Verification items for the finished model (mm, model axes). A direction names the side the tool comes from. Give positions to 0.01 mm unless a question says otherwise; leave off trailing zeros. Order: outer loops, then holes, each group sorted by start corner. A loop starts at its lowest first (then second) coordinate and runs counter-clockwise, first axis right, second up. Notation, with made-up numbers: (62, 82.25) -> (104, 82.25) arc R14 ccw to (104, 106.25) -> close; hole circle Ø5 at (61, 42). An arc over 180 degrees is marked (long way). Return JSON: item names as keys, results as strings. Group by question number.
(1) Cross-section at A-A on x = 17.5. Enter the section's corners in (y, z).
(2) Cross-section at B-B on y = 8. Enter the section's corners in (x, z).
(3) Thickness scan on line 1 along Z through (x, y) = (18.5, 10); line 2 along Z through (x, y) = (16, -9). Record the ranges inside material, lowest first.
(4) Tool access check on faces 1 (the face through (0, 3.134, 61)), 2 (the face through (0, -3.134, 61)), 3 (the face through (0, -18.474, 1)). Record the directions out of +Z, -Z, +X, -X, +Y, -Y that give a thin tool (end or side, any length) a straight path to the whole face; none if there is none.
(5) Depth check by flat-ended pin: pin 1 Ø8 at (y, z) = (12, 54) entering from +X; pin 2 Ø5 at (x, z) = (-4, 40.5) entering from +Y; pin 3 Ø14 at (x, z) = (-11, 60.5) entering from +Y; pin 4 Ø14 at (x, z) = (1.5, 60) entering from -Y. Enter the tip coordinate at first touch or a pass-through.
(6) Cross-section at C-C on z = 41. Enter the section's corners in (x, y), then the cut area to 3 significant figures.
from build123d import *

# Parameters (mm, degrees)
F1_DEPTH      = 25.4
F1_DEPTH_BACK = 25.4


with BuildPart() as f1:
    # F0 (on Right) → F1 (new body, two sides)
    with BuildSketch(Plane.YZ) as f1_sk:
        Polygon((-18.474095, -38.079124), (18.474095, -38.079124), (18.474095, 38.079124), (3.134074, 54.85357), (3.134074, 67.459583), (0, 67.459583), (-3.134074, 67.459583), (-3.134074, 54.85357), (-18.474095, 38.079124), align=None)
    extrude(amount=F1_DEPTH)
    extrude(f1_sk.sketch, amount=-F1_DEPTH_BACK)


solid = f1.part
Verdict:
{
 "1": {"outline": "(-18.47, -38.08) -> (18.47, -38.08) -> (18.47, 38.08) -> (3.13, 54.85) -> (3.13, 67.46) -> (-3.13, 67.46) -> (-3.13, 54.85) -> (-18.47, 38.08) -> close"},
 "2": {"outline": "(-25.4, -38.08) -> (25.4, -38.08) -> (25.4, 49.53) -> (-25.4, 49.53) -> close"},
 "3": {"line 1": "-38.08 to 47.35", "line 2": "-38.08 to 48.44"},
 "4": {"face 1": "+Z, +X, -X, +Y", "face 2": "+Z, +X, -X, -Y", "face 3": "+Z, -Z, +X, -X, -Y"},
 "5": {"pin 1": "through", "pin 2": "y = 18.47", "pin 3": "y = 4.37", "pin 4": "y = -4.83"},
 "6": {"outline": "(-25.4, -15.8) -> (25.4, -15.8) -> (25.4, 15.8) -> (-25.4, 15.8) -> close", "area": "1,610 mm²"}
}
